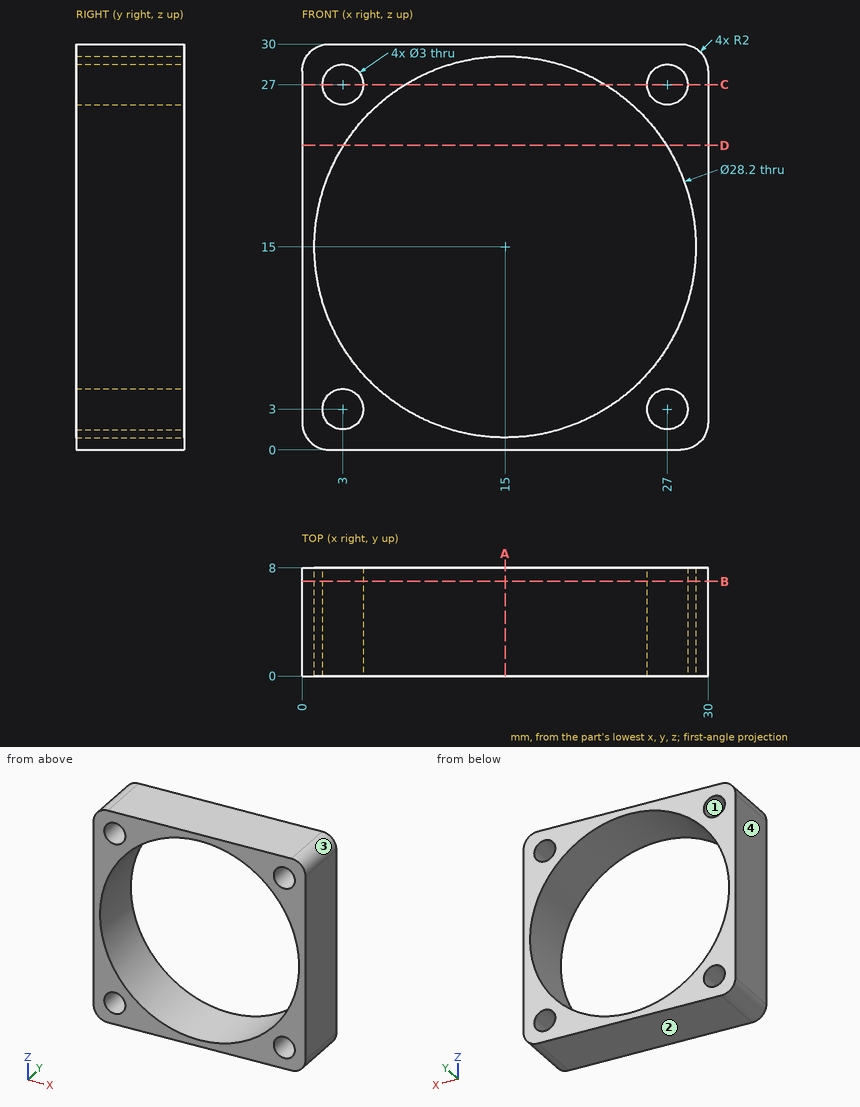
The drawing under review shows one solid part. Ordinate dimensions are in mm from its lowest x, y, z. Give positions to 0.01 mm unless a question says otherwise; leave off trailing zeros. Write each loop counter-clockwise with the first axis right and the second up, starting at its lowest first coordinate (ties: lowest second). Pieces come first, ordered by that corner, then holes. Notation, with made-up numbers: (40.25, 2) - (78.25, 2) arc R20 ccw to (78.25, 9) - close; hole circle Ø8 at (14, 41.25). An arc over 180 degrees is marked (long way). Answer in a Markdown table with one row per item. Add a question column.
1. Insertion check: P1, Ø2.5, axis at x = 3, z = 27, coming from the +Y side. The pin has a flat end and moves straight along its axis. Give the tip position at first contact, or say it passes through.
2. We need section B-B on y = 7. Write out the cut boundary in (x, z).
3. We need section D-D on z = 22.5. Write out the cut boundary in (x, y).
4. Wall thickness on line 1 along X through (y, z) = (5.75, 3); line 2 along Z through (x, y) = (27.25, 4.25); line 3 along Z through (x, y) = (15, 5.25): over which ranges is each line inside the solid? List them lowest first. Write a range as [from, to].
5. Draft analysis for pull direction X (two halves, no side actions). For the marked faces 1, 2, 3 and 4, state which applies: +X half, -X half, draft (parallel to the pull), parting line (faces both ways), or undercut.
6. We need section A-A on x = 15. Write out the cut boundary in (y, z), then the cut area to 3 significant figures.
7. We need section C-C on z = 27. Write out the cut boundary in (x, y), then the cut area to 3 significant figures.
Ans:
| question | item | result |
|---|---|---|
| 1 | P1 | passes through |
| 2 | outline | (0, 2) arc R2 ccw to (2, 0) - (28, 0) arc R2 ccw to (30, 2) - (30, 28) arc R2 ccw to (28, 30) - (2, 30) arc R2 ccw to (0, 28) - close; hole circle Ø28.2 at (15, 15); hole circle Ø3 at (3, 3); hole circle Ø3 at (3, 27); hole circle Ø3 at (27, 3); hole circle Ø3 at (27, 27) |
| 3 | outline | (0, 0) - (3.06, 0) - (3.06, 8) - (0, 8) - close; (26.94, 0) - (30, 0) - (30, 8) - (26.94, 8) - close |
| 4 | line 1 | x = [0, 1.5], [4.5, 7.6], [22.4, 25.5], [28.5, 30] |
| 4 | line 2 | z = [0, 1.52], [4.48, 8.02], [21.98, 25.52], [28.48, 30] |
| 4 | line 3 | z = [0, 0.9], [29.1, 30] |
| 5 | face 1 | undercut |
| 5 | face 2 | draft |
| 5 | face 3 | +X half |
| 5 | face 4 | -X half |
| 6 | outline | (0, 0) - (8, 0) - (8, 0.9) - (0, 0.9) - close; (0, 29.1) - (8, 29.1) - (8, 30) - (0, 30) - close |
| 6 | area | 14.4 mm^2 |
| 7 | outline | (0, 0) - (1.5, 0) - (1.5, 8) - (0, 8) - close; (4.5, 0) - (7.6, 0) - (7.6, 8) - (4.5, 8) - close; (22.4, 0) - (25.5, 0) - (25.5, 8) - (22.4, 8) - close; (28.5, 0) - (30, 0) - (30, 8) - (28.5, 8) - close |
| 7 | area | 73.5 mm^2 |
